Can you work these out from the model? Positions are in its coordinate system, mm. Round coordinates to 2 decimals unless told otherwise and drop trailing zeros. Loops run counter-clockwise (first coordinate to the right, second up) from the corner with the lowest first, then second, coordinate; pieces in that order, holes last. Notation, with made-up numbers: M 17.25,60 L 68.25,60 A24 cw 68.25,78 Z; hole C -35.75,77 d7. An arc over 180 degrees is marked long. Return JSON: item names as keys, results as strings.
```python
from build123d import *

# Parameters (mm, degrees)
BOSS_EXTRUDE1_DEPTH = 5
SKETCH3_R           = 1.85399934
CUT_EXTRUDE1_DEPTH  = 10


with BuildPart() as part:
    # Sketch1 → Boss-Extrude1 (new body)
    with BuildSketch(Plane(origin=(0, 0, 0), x_dir=(1, 0, 0), z_dir=(0, 1, 0))):
        Polygon((-42.454197946, 56.361544115), (-42.454197946, 51.361544115), (-72.454197946, 51.361544115), (-72.454197946, 31.361544115), (-67.454197946, 31.361544115), (-67.454197946, 1.361544115), (-72.454197946, 1.361544115), (-72.454197946, -63.638455885), (-67.454197946, -63.638455885), (-67.454197946, -93.638455885), (-72.454197946, -93.638455885), (-72.454197946, -118.638455885), (-42.454197946, -118.638455885), (-42.454197946, -123.638455885), (-12.454197946, -123.638455885), (-12.454197946, -118.638455885), (32.545802054, -118.638455885), (32.545802054, -123.638455885), (62.545802054, -123.638455885), (62.545802054, -118.638455885), (92.545802054, -118.638455885), (92.545802054, -93.638455885), (87.545802054, -93.638455885), (87.545802054, -63.638455885), (92.545802054, -63.638455885), (92.545802054, 1.361544115), (87.545802054, 1.361544115), (87.545802054, 31.361544115), (92.545802054, 31.361544115), (92.545802054, 51.361544115), (62.545802054, 51.361544115), (62.545802054, 56.361544115), (32.545802054, 56.361544115), (32.545802054, 51.361544115), (-12.454197946, 51.361544115), (-12.454197946, 56.361544115), align=None)
    extrude(amount=BOSS_EXTRUDE1_DEPTH)

    # Sketch3 → Cut-Extrude1 (cut)
    with BuildSketch(Plane(origin=(0, 5, 0), x_dir=(1, 0, 0), z_dir=(0, 1, 0))):
        Polygon((87.295802054, -48.920455885), (87.295802054, -36.455455885), (67.295802054, -36.455455885), (67.295802054, -11.455455885), (-47.136197946, -11.455455885), (-47.136197946, -36.455455885), (-67.136197946, -36.455455885), (-67.136197946, -49.301455885), (-53.721197946, -62.716455885), (-37.879197946, -62.716455885), (-37.879197946, -78.558455885), (-37.799197946, -78.638455885), (57.577802054, -78.638455885), (59.689802054, -76.526455885), (59.689802054, -62.335455885), (73.880802054, -62.335455885), align=None)
        with Locations(Location((-42.879197946, -67.716455885, 0), (0, 0, 270))):
            Circle(SKETCH3_R)
        with Locations(Location((-55.960197946, -17.805455885, 0), (0, 0, 270))):
            Circle(SKETCH3_R)
        with Locations(Location((-55.833197946, -28.981455885, 0), (0, 0, 270))):
            Circle(SKETCH3_R)
        with Locations(Location((64.689802054, -67.335455885, 0), (0, 0, 270))):
            Circle(SKETCH3_R)
        with Locations(Location((74.976802054, -18.186455885, 0), (0, 0, 270))):
            Circle(SKETCH3_R)
        with Locations(Location((74.976802054, -28.854455885, 0), (0, 0, 270))):
            Circle(SKETCH3_R)
    extrude(amount=-CUT_EXTRUDE1_DEPTH, mode=Mode.SUBTRACT)


solid = part.part
```
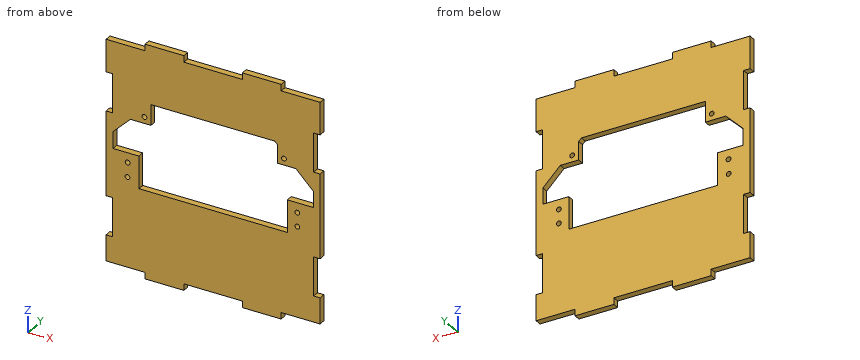
Q1. If I drill on line 1 along Z through (x, y) = (64.5, 0.8); line 2 along Z through (x, y) = (-11.5, 4.45); line 3 along Z through (x, y) = (-49, 3.8), over which ranges is the centre line in solid material (lowest first)?
Results:
{"line 1": "z = -51.36 to 11.46, 62.34 to 65.49, 69.18 to 118.64", "line 2": "z = -51.36 to 11.46, 78.64 to 118.64", "line 3": "z = -51.36 to 36.46, 62.72 to 118.64"}
Q2. Suppose I cut it at A-A, the plane x = -5.5. Please give me the cut outline in (y, z), plus the area to 3 significant figures.
Results:
{"outline": "M 0,-51.36 L 5,-51.36 L 5,11.46 L 0,11.46 Z; M 0,78.64 L 5,78.64 L 5,118.64 L 0,118.64 Z", "area": "514 mm2"}
Q3. Suppose I cut it at B-B, the plane x = 36. Please give me the cut outline in (y, z), plus the area to 3 significant figures.
Results:
{"outline": "M 0,-56.36 L 5,-56.36 L 5,11.46 L 0,11.46 Z; M 0,78.64 L 5,78.64 L 5,123.64 L 0,123.64 Z", "area": "564 mm2"}
Q4. I'm going to push flat-ended pins straight in: pin 1 Ø10 at (x, z) = (-51, -3.5) entering from -Y; pin 2 Ø1.5 at (x, y) = (-1.5, 2.5) entering from +Z; pin 3 Ø3 at (y, z) = (1, -25) entering from -X; pin 4 Ø2.5 at (x, y) = (89, 2) entering from -Z. Where does each tip first touch, or does it pass through?
Results:
{"pin 1": "stops at y = 0", "pin 2": "stops at z = 118.64", "pin 3": "stops at x = -67.45", "pin 4": "stops at z = -51.36"}
Q5. Suppose I cut it at D-D, the plane y = 3.1. State how many separate pieces and enclosed holes the cut face has, plus the area to 3 significant figures.
Results:
{"separate pieces": "1", "enclosed holes": "7", "area": "19,700 mm2"}
Q6. Suppose I cut it at C-C, the plane z = -27.5. Please give me the cut outline in (x, y), plus the area to 3 significant figures.
Results:
{"outline": "M -67.45,0 L 87.55,0 L 87.55,5 L -67.45,5 Z", "area": "775 mm2"}
